```python
from build123d import *

# Parameters (mm, degrees)
SKETCH1_W           = 132
SKETCH1_H           = 100
BOSS_EXTRUDE1_DEPTH = 5
SKETCH2_R           = 1.75
CUT_EXTRUDE1_DEPTH  = 56
CUT_EXTRUDE4_DEPTH  = 103
SKETCH4_R           = 1.75
CUT_EXTRUDE5_DEPTH  = 103
SKETCH6_R           = 3.5
CUT_EXTRUDE6_DEPTH  = 3
CUT_EXTRUDE7_DEPTH  = 3.5


with BuildPart() as part:
    # Sketch1 → Boss-Extrude1 (new body)
    with BuildSketch(Plane(origin=(0, 0, 0), x_dir=(1, 0, 0), z_dir=(0, 1, 0))):
        Rectangle(SKETCH1_W, SKETCH1_H)
    extrude(amount=BOSS_EXTRUDE1_DEPTH)

    # Sketch2 → Cut-Extrude1 (cut)
    with BuildSketch(Plane(origin=(0, 5, 0), x_dir=(1, 0, 0), z_dir=(0, 1, 0))):
        with Locations(Location((-59.5, 34.72, 0), (0, 0, 270))):
            Circle(SKETCH2_R)
        with Locations(Location((-59.5, -40.36, 0), (0, 0, 270))):
            Circle(SKETCH2_R)
        with Locations(Location((59.5, -40.36, 0), (0, 0, 270))):
            Circle(SKETCH2_R)
        with Locations(Location((59.5, 34.72, 0), (0, 0, 270))):
            Circle(SKETCH2_R)
    extrude(amount=-CUT_EXTRUDE1_DEPTH, mode=Mode.SUBTRACT)

    # Sketch3 → Cut-Extrude4 (cut)
    with BuildSketch(Plane(origin=(0, 5, 0), x_dir=(1, 0, 0), z_dir=(0, 1, 0))):
        Polygon((-17.5, 50), (17.5, 50), (17.5, 16.5), (47.5, 16.5), (47.5, -28.5), (-47.5, -28.5), (-47.5, 16.5), (-17.5, 16.5), align=None)
    extrude(amount=-CUT_EXTRUDE4_DEPTH, mode=Mode.SUBTRACT)

    # Sketch4 → Cut-Extrude5 (cut)
    with BuildSketch(Plane(origin=(0, 5, 0), x_dir=(1, 0, 0), z_dir=(0, 1, 0))):
        with Locations(Location((-28.5, 22, 0), (0, 0, 270))):
            Circle(SKETCH4_R)
        with Locations(Location((-28.5, -35, 0), (0, 0, 270))):
            Circle(SKETCH4_R)
        with Locations(Location((28.5, -35, 0), (0, 0, 270))):
            Circle(SKETCH4_R)
        with Locations(Location((28.5, 22, 0), (0, 0, 270))):
            Circle(SKETCH4_R)
    extrude(amount=-CUT_EXTRUDE5_DEPTH, mode=Mode.SUBTRACT)

    # Sketch6 → Cut-Extrude6 (cut)
    with BuildSketch(Plane(origin=(0, 5, 0), x_dir=(1, 0, 0), z_dir=(0, 1, 0))):
        with Locations(Location((-59.5, 34.72, 0), (0, 0, 270))):
            Circle(SKETCH6_R)
        with Locations(Location((-59.5, -40.36, 0), (0, 0, 270))):
            Circle(SKETCH6_R)
        with Locations(Location((59.5, -40.36, 0), (0, 0, 270))):
            Circle(SKETCH6_R)
        with Locations(Location((59.5, 34.72, 0), (0, 0, 270))):
            Circle(SKETCH6_R)
    extrude(amount=-CUT_EXTRUDE6_DEPTH, mode=Mode.SUBTRACT)

    # Sketch7 → Cut-Extrude7 (cut)
    with BuildSketch(Plane.XZ):
        Polygon((26.479274058, -25.5), (30.520725942, -25.5), (32.541451884, -22), (30.520725942, -18.5), (26.479274058, -18.5), (24.458548116, -22), align=None)
        Polygon((24.458548116, 35), (26.479274058, 31.5), (30.520725942, 31.5), (32.541451884, 35), (30.520725942, 38.5), (26.479274058, 38.5), align=None)
        Polygon((-30.520725942, 38.5), (-32.541451884, 35), (-30.520725942, 31.5), (-26.479274058, 31.5), (-24.458548116, 35), (-26.479274058, 38.5), align=None)
        Polygon((-32.541451884, -22), (-30.520725942, -25.5), (-26.479274058, -25.5), (-24.458548116, -22), (-26.479274058, -18.5), (-30.520725942, -18.5), align=None)
    extrude(amount=-CUT_EXTRUDE7_DEPTH, mode=Mode.SUBTRACT)


solid = part.part
```
Geometry: final body of the model. Coordinates: model frame, mm. A direction names the side the tool comes from. Round coordinates to 2 decimals unless told otherwise and drop trailing zeros. Order: outer loops, then holes, each group sorted by start corner. A loop starts at its lowest first (then second) coordinate and runs counter-clockwise, first axis right, second up. Notation, with made-up numbers: M 55,-30.5 L 67,-30.5 A5 ccw 67,-22.5 Z; hole C 78,67 d10. An arc over 180 degrees is marked long. One line per item, written item: value.
(1) Cut plane C-C (x = -36). Return the cut outline in (y, z).
Result sheet:
outline: M 0,-50 L 5,-50 L 5,-16.5 L 0,-16.5 Z; M 0,28.5 L 5,28.5 L 5,50 L 0,50 Z
(2) Cut plane D-D (x = 28.5). Return the cut outline in (y, z), and give its area (4 significant figures).
Result sheet:
outline: M 0,-50 L 5,-50 L 5,-23.75 L 3.5,-23.75 L 3.5,-25.5 L 0,-25.5 Z; M 0,-18.5 L 3.5,-18.5 L 3.5,-20.25 L 5,-20.25 L 5,-16.5 L 0,-16.5 Z; M 0,28.5 L 5,28.5 L 5,33.25 L 3.5,33.25 L 3.5,31.5 L 0,31.5 Z; M 0,38.5 L 3.5,38.5 L 3.5,36.75 L 5,36.75 L 5,50 L 0,50 Z
area: 215.5 mm2
(3) Reachability of faces 5 (the flat face through (31.5, 1.7, 33.2)), 6 (the flat face through (1, 3, 28.5)), 7 (the flat face through (-66, 2, 1)) from +Z, -Z, +X, -X, +Y, -Y: full face, straight path, thin tool, end or side. Return the list, or none.
Result sheet:
face 5: -Y
face 6: +Y, -Y
face 7: +Z, -Z, -X, +Y, -Y
(4) Pin query (flat end, axial travel): P1, Ø4, axis at x = 59.5, z = 40.36, coming from the -Y side; P2, Ø2, axis at x = 58.5, z = 40, coming from the +Y side. Return the tip coordinate at first contact, or that it passes through.
Result sheet:
P1: y = 0
P2: y = 2
(5) Cut plane B-B (z = -34.72). Return the cut outline in (x, y), and give its area (3 significant figures).
Result sheet:
outline: M -66,0 L -61.25,0 L -61.25,2 L -63,2 L -63,5 L -66,5 Z; M -57.75,0 L -17.5,0 L -17.5,5 L -56,5 L -56,2 L -57.75,2 Z; M 17.5,0 L 57.75,0 L 57.75,2 L 56,2 L 56,5 L 17.5,5 Z; M 61.25,0 L 66,0 L 66,5 L 63,5 L 63,2 L 61.25,2 Z
area: 429 mm2
(6) Pull-direction query (X, two-part tool) for faces 1 (the flat face through (66, 2, 1)), 2 (the flat face through (-1, 5, 33)), 3 (the flat face through (61, 2, -36)), 4 (the flat face through (25.5, 1.7, 36.8)); classes: pulls with the +X half, pulls with the -X half, needs draft (parallel to the pull), parting line crosses it, or undercut.
Result sheet:
face 1: pulls with the +X half
face 2: needs draft
face 3: undercut
face 4: undercut
(7) Cut plane A-A (z = 40.36). Return the cut outline in (x, y), and give its area (3 significant figures).
Result sheet:
outline: M -66,0 L -61.25,0 L -61.25,2 L -63,2 L -63,5 L -66,5 Z; M -57.75,0 L 57.75,0 L 57.75,2 L 56,2 L 56,5 L -56,5 L -56,2 L -57.75,2 Z; M 61.25,0 L 66,0 L 66,5 L 63,5 L 63,2 L 61.25,2 Z
area: 604 mm2
(8) Line query: probe 1 along X at (y, z) = (4.45, 40.36); probe 2 along X at (y, z) = (2.2, -35); probe 3 along X at (y, z) = (3.3, 16). Output: solid intervals per line, ascending. Write a range as [from, to].
Result sheet:
probe 1: [-66, -63], [-56, 56], [63, 66]
probe 2: [-66, -62.99], [-56.01, -17.5], [17.5, 56.01], [62.99, 66]
probe 3: [-66, -47.5], [47.5, 66]
